from build123d import *

# Parameters (mm, degrees)
BOSS_EXTRUDE1_DEPTH = 38.1
CUT_EXTRUDE1_DEPTH  = 30.48


with BuildPart() as part:
    # Sketch1 → Boss-Extrude1 (new body)
    with BuildSketch(Plane(origin=(0, 0, 0), x_dir=(1, 0, 0), z_dir=(0, 1, 0))):
        Polygon((-0.111992667, 54.937923296), (-38.926168882, 38.767787333), (-54.937923296, -0.111992667), (-38.767787333, -38.926168882), (0.111992667, -54.937923296), (38.926168882, -38.767787333), (54.937923296, 0.111992667), (38.767787333, 38.926168882), align=None)
    extrude(amount=BOSS_EXTRUDE1_DEPTH)

    # Sketch2 → Cut-Extrude1 (cut)
    with BuildSketch(Plane(origin=(0, 38.1, 0), x_dir=(1, 0, 0), z_dir=(0, 1, 0))):
        Polygon((16.590278128, -10.100852389), (-4.511730777, -18.892030932), (14.673385048, -48.8715909), (24.364776501, -44.834119729), align=None)
        Polygon((-10.100852389, -16.590278128), (-18.892030932, 4.511730777), (-48.8715909, -14.673385048), (-44.834119729, -24.364776501), align=None)
        Polygon((-16.590278128, 10.100852389), (4.511730777, 18.892030932), (-14.673385048, 48.8715909), (-24.364776501, 44.834119729), align=None)
        Polygon((10.100852389, 16.590278128), (18.892030932, -4.511730777), (48.8715909, 14.673385048), (44.834119729, 24.364776501), align=None)
    extrude(amount=-CUT_EXTRUDE1_DEPTH, mode=Mode.SUBTRACT)


solid = part.part
For this review, take the finished solid that the model builds, in its own axes (mm). A direction names the side the tool comes from. Give positions to 0.01 mm unless a question says otherwise; leave off trailing zeros. Order: outer loops, then holes, each group sorted by start corner. A loop starts at its lowest first (then second) coordinate and runs counter-clockwise, first axis right, second up. Notation, with made-up numbers: (47, 19.5) - (95, 19.5) arc R20 ccw to (95, 51.5) - close; hole circle Ø6 at (23.5, 51). An arc over 180 degrees is marked (long way). Answer as a JSON object with one key per item and string values. Group by question number.
Item 1: Wall thickness on line 1 along Z through (x, y) = (-1, 13); line 2 along Z through (x, y) = (0, 25.5); line 3 along Y through (x, z) = (-8, -15): over which ranges is each line inside the solid? List them lowest first.
Item 2: Take a section at A-A on y = 3.5. Give the boundary of the cut face in (x, z), and give its area (3 significant figures).
Item 3: Clearance check with flat-ended pins moving along their axes: pin 1 Ø5 at (x, y) = (8.5, 28.5) entering from +Z; pin 2 Ø2 at (y, z) = (16, -3.5) entering from +X; pin 3 Ø2 at (y, z) = (22.5, 36) entering from -X. State where each tip first meets the part, or that it passes through.
Item 4: Take a section at D-D on y = 34.5. Give the boundary of the cut face in (x, z).
Item 5: Take a section at C-C on z = -36.5. Give the boundary of the cut face in (x, y).
Item 6: Machinability: for faces 1 (the flat face through (-43.373, 18.783, 27.873)), 2 (the flat face through (13, 7.62, 29)), 3 (the flat face through (-20.53, 23.07, -27.71)), which of the approach directions +Z, -Z, +X, -X, +Y, -Y give a long, thin tool a straight path to every point of the face, cutting with its end or side? Answer none if there is none.
Item 7: Take a section at B-B on x = -11.5. Give the boundary of the cut face in (y, z), and give its area (3 significant figures).
Item 8: Draft analysis for pull direction Z (two halves, no side actions). For faces 4 (the flat face through (-27.71, 23.07, 20.53)), 5 (the flat face through (-27.873, 18.783, -43.373)), 6 (the flat face through (46.82, 18.78, 19.6)), 7 (the flat face through (27.71, 23.07, -20.53)), state which applies: pulls with the +Z half, pulls with the -Z half, needs draft (parallel to the pull), parting line crosses it, or undercut.
Reported:
{
 "1": {"line 1": "-54.57 to -27.5, -16.6 to 17.43, 24.38 to 54.48", "line 2": "-54.89 to -25.94, -17.01 to 17.01, 25.94 to 54.89", "line 3": "0 to 7.62"},
 "2": {"outline": "(-54.94, 0.11) - (-38.93, -38.77) - (-0.11, -54.94) - (38.77, -38.93) - (54.94, -0.11) - (38.93, 38.77) - (0.11, 54.94) - (-38.77, 38.93) - close", "area": "8,540 mm^2"},
 "3": {"pin 1": "z = 52.48", "pin 2": "x = 53.94", "pin 3": "x = -40.4"},
 "4": {"outline": "(-54.94, 0.11) - (-38.93, -38.77) - (-24.36, -44.83) - (-16.59, -10.1) - (4.51, -18.89) - (-14.67, -48.87) - (-0.11, -54.94) - (38.77, -38.93) - (44.83, -24.36) - (10.1, -16.59) - (18.89, 4.51) - (48.87, -14.67) - (54.94, -0.11) - (38.93, 38.77) - (24.36, 44.83) - (16.59, 10.1) - (-4.51, 18.89) - (14.67, 48.87) - (0.11, 54.94) - (-38.77, 38.93) - (-44.83, 24.36) - (-10.1, 16.59) - (-18.89, -4.51) - (-48.87, 14.67) - close"},
 "5": {"outline": "(-39.86, 0) - (39.78, 0) - (39.78, 38.1) - (-6.76, 38.1) - (-6.76, 7.62) - (-22.5, 7.62) - (-22.5, 38.1) - (-39.86, 38.1) - close"},
 "6": {"face 1": "+Z, -X, +Y, -Y", "face 2": "+Y", "face 3": "-Z, +Y"},
 "7": {"outline": "(0, -50.19) - (38.1, -50.19) - (38.1, -43.91) - (7.62, -43.91) - (7.62, -12.22) - (38.1, -12.22) - (38.1, 13.23) - (7.62, 13.23) - (7.62, 16.9) - (38.1, 16.9) - (38.1, 50.16) - (0, 50.16) - close", "area": "2,750 mm^2"},
 "8": {"face 4": "undercut", "face 5": "pulls with the -Z half", "face 6": "pulls with the +Z half", "face 7": "undercut"}
}
